Answer from the drawing. Dimensions are ordinates in mm from the lowest x, y and z of the part. Give positions to 0.01 mm unless a question says otherwise; leave off trailing zeros. Loops run counter-clockwise (first coordinate to the right, second up) from the corner with the lowest first, then second, coordinate; pieces in that order, holes last. Notation, with made-up numbers: (61.25, 45.5) - (74.25, 45.5) arc R22 cw to (74.25, 74.5) - close; hole circle Ø10 at (75.25, 17). An arc over 180 degrees is marked (long way). Answer as CSV lines item,"result". Start each with the question number.
1) A cutting plane is placed at C-C (y = 44.5). Determine the outline of the cut face in (x, z).
2) Find the intervals of material crossed by line 1 along X through (y, z) = (31.5, 3.4); line 2 along Y through (x, z) = (34, 1.6); line 3 along Y through (x, z) = (5, 2.2), in increasing order.
3) A cutting plane is placed at A-A (x = 5). Determine the outline of the cut face in (y, z), and give its area (3 significant figures).
4) For a pull along X with two mould halves and no side action, classify the marked faces 1 and 2 as pulls with the +X half, pulls with the -X half, needs draft (parallel to the pull), parting line crosses it, or undercut.
5) Flat-ended cylindrical pins translate along their axes: pin 1 (1 mm diameter, centred on y = 21, z = 4, fed in from +X); pin 2 (1.5 mm diameter, centred on y = 22.5, z = 2.5, fed in from +X). Find the tip coordinate at first contact, or state that the pin passes through.
6) A cutting plane is placed at B-B (z = 4.3). Determine the outline of the cut face in (x, y).
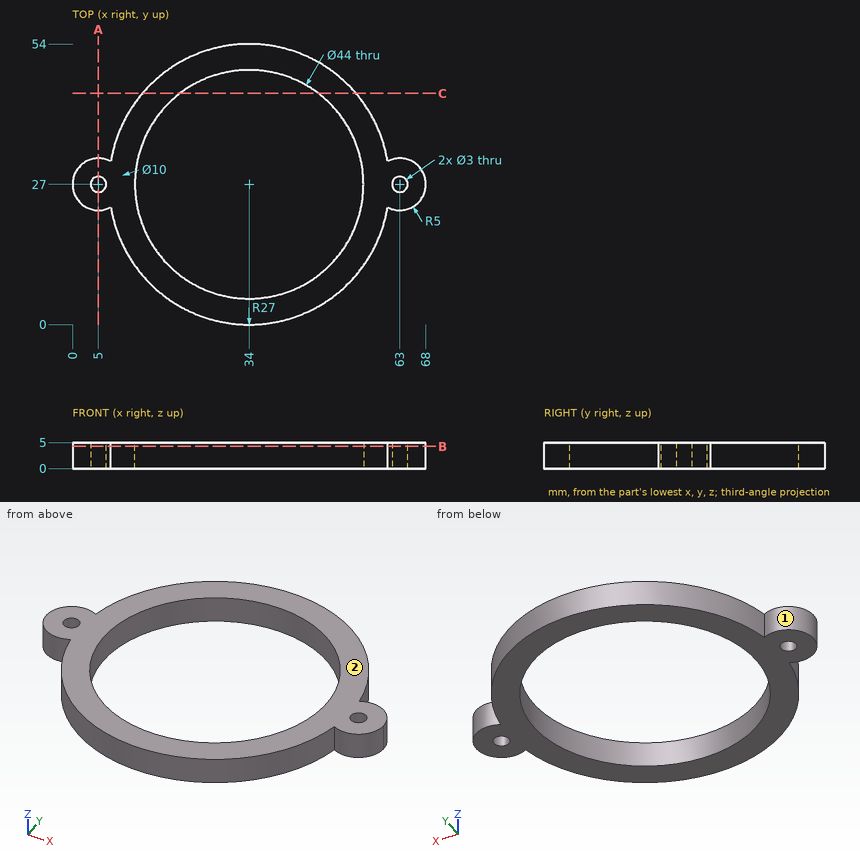
Ans:
1,outline,"(13.44, 0) - (20.67, 0) - (20.67, 5) - (13.44, 5) - close; (47.33, 0) - (54.56, 0) - (54.56, 5) - (47.33, 5) - close"
2,line 1,"2.82 to 7.18, 7.38 to 12.47, 55.53 to 60.62, 60.82 to 65.18"
2,line 2,"0 to 5, 49 to 54"
2,line 3,"22 to 25.5, 28.5 to 32"
3,outline,"(22, 0) - (25.5, 0) - (25.5, 5) - (22, 5) - close; (28.5, 0) - (32, 0) - (32, 5) - (28.5, 5) - close"
3,area,"35.0 mm2"
4,face 1,"undercut"
4,face 2,"needs draft"
5,pin 1,"x = 60.43"
5,pin 2,"x = 66.31"
6,outline,"(7.36, 22.59) arc R27 ccw to (60.64, 22.59) arc R5 ccw (long way) to (60.64, 31.41) arc R27 ccw to (7.36, 31.41) arc R5 ccw (long way) to start; hole circle Ø3 at (5, 27); hole circle Ø44 at (34, 27); hole circle Ø3 at (63, 27)"
